The listing builds one solid part. Answer for the finished solid, in the listing's coordinates (mm). Face numbers are marked on the shaded views. A direction names the side the tool comes from. Coordinates: 2 decimals unless noted, no trailing zeros. Loops run counter-clockwise (first coordinate to the right, second up) from the corner with the lowest first, then second, coordinate; pieces in that order, holes last. Notation, with made-up numbers: (36, 70.5) -> (70, 70.5) arc R27 cw to (70, 94.5) -> close; hole circle Ø2 at (-9.75, 8). An arc over 180 degrees is marked (long way). Answer in a Markdown table with one row per item.
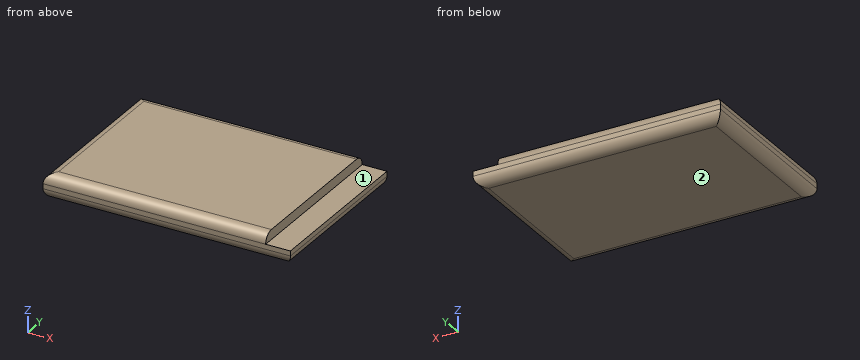
```python
from build123d import *

# Parameters (mm, degrees)
F0_W     = 50
F0_H     = 34
F1_DEPTH = 5
F2_W     = 5
F2_H     = 34
F3_DEPTH = 2
F4_R     = 2


with BuildPart() as f1:
    # F0 (on Top) → F1 (new body)
    with BuildSketch(Plane.XY):
        Rectangle(F0_W, F0_H)
    extrude(amount=F1_DEPTH)

    # F2 (on face) → F3 (cut)
    with BuildSketch(Plane.XY.offset(5)):
        with Locations((22.5, 0)):
            Rectangle(F2_W, F2_H)
    extrude(amount=-F3_DEPTH, mode=Mode.SUBTRACT)

    # F4
    f4_edges = [f1.edges().sort_by_distance(p)[0] for p in [
        (-2.5, 17, 5),
        (-2.5, -17, 5),
        (0, -17, 0),
        (0, 17, 0),
        (-25, 0, 0),
        (-25, 0, 5),
        (25, 0, 0),
    ]]
    fillet(f4_edges, radius=F4_R)


solid = f1.part
```
Item 1: A tool of negligible diameter and unlimited length cuts with its end or side. For the marked faces 1 and 2, from which of +Z, -Z, +X, -X, +Y, -Y can it reach the whole face along a straight path? Write none if from no direction.
Findings below:
| item | result |
|---|---|
| face 1 | +Z, +X, +Y, -Y |
| face 2 | -Z, +X, -X, +Y, -Y |
Item 2: A cutting plane is placed at C-C, the plane z = 3.65. Determine the outline of the cut face in (x, y), plus the area to 3 significant figures.
Findings below:
| item | result |
|---|---|
| outline | (-24.89, -16.89) -> (20, -16.89) -> (20, 16.89) -> (-24.89, 16.89) -> close |
| area | 1,520 mm2 |
Item 3: A cutting plane is placed at D-D, the plane z = 1.1. Determine the outline of the cut face in (x, y).
Findings below:
| item | result |
|---|---|
| outline | (-24.79, -16.79) -> (24.79, -16.79) -> (24.79, 16.79) -> (-24.79, 16.79) -> close |
Item 4: Flat-ended cylindrical pins translate along their axes: pin 1 Ø1.5 at (x, y) = (21.5, -0.5) entering from +Z; pin 2 Ø1.6 at (y, z) = (-6.5, 4) entering from +X. Find the tip coordinate at first contact, or state that the pin passes through.
Findings below:
| item | result |
|---|---|
| pin 1 | stops at z = 3 |
| pin 2 | stops at x = 20 |
Item 5: A cutting plane is placed at B-B, the plane y = 13. Determine the outline of the cut face in (x, z), plus the area to 3 significant figures.
Findings below:
| item | result |
|---|---|
| outline | (-25, 2) arc R2 ccw to (-23, 0) -> (23, 0) arc R2 ccw to (25, 2) -> (25, 3) -> (20, 3) -> (20, 5) -> (-23, 5) arc R2 ccw to (-25, 3) -> close |
| area | 237 mm2 |
Item 6: A cutting plane is placed at A-A, the plane x = -12. Determine the outline of the cut face in (y, z), plus the area to 3 significant figures.
Findings below:
| item | result |
|---|---|
| outline | (-17, 2) arc R2 ccw to (-15, 0) -> (15, 0) arc R2 ccw to (17, 2) -> (17, 3) arc R2 ccw to (15, 5) -> (-15, 5) arc R2 ccw to (-17, 3) -> close |
| area | 167 mm2 |
Item 7: Find the intervals of material crossed by probe 1 along X at (y, z) = (-15, 1.85); probe 2 along Z at (x, y) = (22.5, -6.5); probe 3 along X at (y, z) = (-14, 3.95), in increasing order.
Findings below:
| item | result |
|---|---|
| probe 1 | x = -24.99 to 24.99 |
| probe 2 | z = 0 to 3 |
| probe 3 | x = -24.76 to 20 |
